Design review of the part built by this model. Coordinates are the model's own, in mm. A direction names the side the tool comes from. Coordinates: 2 decimals unless noted, no trailing zeros. Loops run counter-clockwise (first coordinate to the right, second up) from the corner with the lowest first, then second, coordinate; pieces in that order, holes last. Notation, with made-up numbers: (-16.75, 15) - (27.25, 15) arc R20 ccw to (27.25, 43) - close; hole circle Ø6 at (21, -12). An arc over 180 degrees is marked (long way). Return JSON: item names as keys, results as strings. Group by question number.
from build123d import *

# Parameters (mm, degrees)
SKETCH1_R                   = 3.175
BOSS_EXTRUDE1_DEPTH         = 12.7
SKETCH3_R                   = 83.82
SKETCH3_R_2                 = 81.9404
CUT_EXTRUDE1_DEPTH          = 6.35
CUT_EXTRUDE2_START          = -6.35
CUT_EXTRUDE2_OUTLINE_R      = 81.9404
CUT_EXTRUDE2_DEPTH          = 6.35
F_1_4_0_25_DIAMETER_HOLE1_D = 6.35
FILLET1_R                   = 6.35
CUT_EXTRUDE3_DEPTH          = 1047.720478305


# Read off the part's stored shape, not the designer's step: Cut-Extrude2
with BuildPart() as part:
    # Sketch1 → Boss-Extrude1 (new body)
    with BuildSketch(Plane.XZ.offset(-27489.985969718)):
        Polygon((556.409465543, 581.693641464), (28.480379396, 886.493641464), (-276.319620604, 358.564555317), (251.609465543, 53.764555317), align=None)
        with Locations((-206.925530091, 377.158645829)):
            Circle(SKETCH1_R, mode=Mode.SUBTRACT)
        with Locations((233.015375031, 123.158645829)):
            Circle(SKETCH1_R, mode=Mode.SUBTRACT)
        with Locations((487.015375031, 563.099550952)):
            Circle(SKETCH1_R, mode=Mode.SUBTRACT)
        with Locations((47.074469909, 817.099550952)):
            Circle(SKETCH1_R, mode=Mode.SUBTRACT)
        with BuildLine():
            Line((-37.632916951, 543.382053135), (-48.631439579, 549.732053135))
            Line((-48.631439579, 549.732053135), (-35.931439579, 571.729098391))
            Line((-35.931439579, 571.729098391), (-13.934394323, 559.029098391))
            Line((-13.934394323, 559.029098391), (-20.284394323, 548.030575763))
            ThreePointArc((-20.284394323, 548.030575763), (-27.995915078, 542.113317769), (-37.632916951, 543.382053135))
        make_face(mode=Mode.SUBTRACT)
        with BuildLine():
            Line((241.64492247, 646.10546044), (263.641967726, 633.40546044))
            Line((263.641967726, 633.40546044), (257.291967726, 622.406937812))
            ThreePointArc((257.291967726, 622.406937812), (249.580446971, 616.489679818), (239.943445098, 617.758415184))
            Line((239.943445098, 617.758415184), (228.94492247, 624.108415184))
            Line((228.94492247, 624.108415184), (241.64492247, 646.10546044))
        make_face(mode=Mode.SUBTRACT)
    extrude(amount=BOSS_EXTRUDE1_DEPTH)

    # Sketch3 → Cut-Extrude1 (cut)
    with BuildSketch(Plane.XZ.offset(-27489.985969718)):
        with Locations((140.04492247, 470.129098391)):
            Circle(SKETCH3_R)
        with Locations((140.04492247, 470.129098391)):
            Circle(SKETCH3_R_2, mode=Mode.SUBTRACT)
    extrude(amount=CUT_EXTRUDE1_DEPTH, mode=Mode.SUBTRACT)

    # Cut-Extrude2 outline → Cut-Extrude2 (cut)
    with BuildSketch(Plane(origin=(0, 27489.985969718, 0), x_dir=(1, 0, 0), z_dir=(0, 1, 0)).offset(CUT_EXTRUDE2_START)):
        with Locations((140.04492247, -470.129098391)):
            Circle(CUT_EXTRUDE2_OUTLINE_R)
        with BuildLine():
            ThreePointArc((74.203873091, -422.730325217), (99.48112247, -399.870535843), (131.916905483, -389.409690429))
            ThreePointArc((131.916905483, -389.409690429), (135.589601797, -390.547508644), (137.326798106, -393.977592825))
            ThreePointArc((137.326798106, -393.977592825), (140.04492247, -396.516851306), (142.763046834, -393.977592825))
            ThreePointArc((142.763046834, -393.977592825), (144.500243143, -390.547508644), (148.172939457, -389.409690429))
            ThreePointArc((148.172939457, -389.409690429), (180.60872247, -399.870535843), (205.885971849, -422.730325217))
            ThreePointArc((205.885971849, -422.730325217), (206.736940528, -426.479882633), (204.634998644, -429.699380858))
            ThreePointArc((204.634998644, -429.699380858), (203.794998475, -433.322974849), (207.353123009, -434.407310358))
            ThreePointArc((207.353123009, -434.407310358), (211.192261201, -434.196724402), (214.013988837, -436.808463603))
            ThreePointArc((214.013988837, -436.808463603), (221.17252247, -470.129098391), (214.013988837, -503.449733178))
            ThreePointArc((214.013988837, -503.449733178), (211.192261202, -506.06147238), (207.353123009, -505.850886424))
            ThreePointArc((207.353123009, -505.850886424), (203.794998475, -506.935221933), (204.634998644, -510.558815924))
            ThreePointArc((204.634998644, -510.558815924), (206.736940528, -513.778314149), (205.885971849, -517.527871565))
            ThreePointArc((205.885971849, -517.527871565), (180.60872247, -540.387660939), (148.172939457, -550.848506352))
            ThreePointArc((148.172939457, -550.848506352), (144.500243143, -549.710688138), (142.763046834, -546.280603957))
            ThreePointArc((142.763046834, -546.280603957), (140.04492247, -543.741345476), (137.326798106, -546.280603957))
            ThreePointArc((137.326798106, -546.280603957), (135.589601797, -549.710688138), (131.916905483, -550.848506352))
            ThreePointArc((131.916905483, -550.848506352), (99.48112247, -540.387660939), (74.203873091, -517.527871565))
            ThreePointArc((74.203873091, -517.527871565), (73.352904412, -513.778314149), (75.454846296, -510.558815924))
            ThreePointArc((75.454846296, -510.558815924), (76.294846465, -506.935221933), (72.736721931, -505.850886424))
            ThreePointArc((72.736721931, -505.850886424), (68.897583739, -506.06147238), (66.075856104, -503.449733178))
            ThreePointArc((66.075856104, -503.449733178), (58.91732247, -470.12909839), (66.075856104, -436.808463603))
            ThreePointArc((66.075856104, -436.808463603), (68.897583739, -434.196724402), (72.736721931, -434.407310358))
            ThreePointArc((72.736721931, -434.407310358), (76.294846465, -433.322974849), (75.454846296, -429.699380858))
            ThreePointArc((75.454846296, -429.699380858), (73.352904412, -426.479882633), (74.203873091, -422.730325217))
        make_face(mode=Mode.SUBTRACT)
    extrude(amount=CUT_EXTRUDE2_DEPTH, mode=Mode.SUBTRACT)

    # 1/4 (0.25) Diameter Hole1 (through all)
    with Locations(Plane(origin=(0, 27477.285969718, 0), x_dir=(-1, 0, 0), z_dir=(0, -1, 0))):
        with Locations((-276.56992247, -706.597334894), (-276.56992247, -233.660861887), (133.00507753, -470.129098391), (-140.04492247, -470.129098391)):
            Hole(F_1_4_0_25_DIAMETER_HOLE1_D / 2)

    # Fillet1
    fillet1_edges = [part.edges().sort_by_distance(p)[0] for p in [
        (-13.934394323, 27483.635969718, 559.029098391),
        (-35.931439579, 27483.635969718, 571.729098391),
        (-48.631439579, 27483.635969718, 549.732053135),
        (241.64492247, 27483.635969718, 646.10546044),
        (228.94492247, 27483.635969718, 624.108415184),
        (263.641967726, 27483.635969718, 633.40546044),
    ]]
    fillet(fillet1_edges, radius=FILLET1_R)

    # Sketch7 → Cut-Extrude3 (cut, through all)
    with BuildSketch(Plane(origin=(0, 27489.985969718, 0), x_dir=(1, 0, 0), z_dir=(0, 1, 0))):
        with BuildLine():
            Line((87.519099271, -555.383941842), (88.589697985, -541.194514974))
            ThreePointArc((88.589697985, -541.194514974), (90.165199445, -538.685494585), (93.125578624, -538.569119019))
            Line((93.125578624, -538.569119019), (98.706273756, -541.238167012))
            ThreePointArc((98.706273756, -541.238167012), (98.923894245, -541.352808536), (99.131986961, -541.483952646))
            Line((99.131986961, -541.483952646), (104.233797894, -544.982452404))
            ThreePointArc((104.233797894, -544.982452404), (105.613203287, -547.604403762), (104.228078621, -550.223338244))
            Line((104.228078621, -550.223338244), (92.474973845, -558.245217361))
            ThreePointArc((92.474973845, -558.245217361), (89.0976004, -558.372448725), (87.519099271, -555.383941842))
        make_face()
        with BuildLine():
            Line((92.474973844, -382.01297942), (104.228078621, -390.034858537))
            ThreePointArc((104.228078621, -390.034858537), (105.613203286, -392.65379302), (104.233797893, -395.275744378))
            Line((104.233797893, -395.275744378), (99.131986961, -398.774244135))
            ThreePointArc((99.131986961, -398.774244135), (98.923894245, -398.905388245), (98.706273756, -399.020029769))
            Line((98.706273756, -399.020029769), (93.125578624, -401.689077763))
            ThreePointArc((93.125578624, -401.689077763), (90.165199444, -401.572702196), (88.589697984, -399.063681808))
            Line((88.589697984, -399.063681808), (87.519099271, -384.874254939))
            ThreePointArc((87.519099271, -384.874254939), (89.0976004, -381.885748056), (92.474973844, -382.01297942))
        make_face()
        with BuildLine():
            Line((240.140694294, -472.990373909), (227.316990804, -479.157921661))
            ThreePointArc((227.316990804, -479.157921661), (224.356364679, -479.048007567), (222.775390892, -476.542431776))
            Line((222.775390892, -476.542431776), (222.296506693, -470.374884024))
            ThreePointArc((222.296506693, -470.374884024), (222.28697892, -470.12909839), (222.296506693, -469.883312757))
            Line((222.296506693, -469.883312757), (222.775390892, -463.715765005))
            ThreePointArc((222.775390892, -463.715765005), (224.356364679, -461.210189214), (227.316990804, -461.10027512))
            Line((227.316990804, -461.10027512), (240.140694294, -467.267822872))
            ThreePointArc((240.140694294, -467.267822872), (241.939566609, -470.12909839), (240.140694294, -472.990373909))
        make_face()
    extrude(amount=-CUT_EXTRUDE3_DEPTH, mode=Mode.SUBTRACT)


solid = part.part
Item 1: Add section C-C (x = 6). State the section outline as (y, z) points.
Item 2: To check wall thickness, follow line 1 (X direction, y = 27483, z = 548); line 2 (X direction, y = 27489.75, z = 440); line 3 (X direction, y = 27478.75, z = 619). State the ranges of each line that lie inside material, in increasing order. Write a range as from..to.
Item 3: Add section A-A (y = 27485.75). Give the number of separate pieces and of enclosed holes in the cut face, then the cut area to 3 significant figures.
Item 4: Add section B-B (z = 140). State the section outline as (x, y) points.
Item 5: For faces 5 (the face through (-16.05, 27483.72, 208.3)), 6 (the face through (180.99, 27486.86, 396.99)), list the 3-axis set-ups (+Z, -Z, +X, -X, +Y, -Y) from which the entire face can be reached by the end or side of a thin tool; tool diameter is ignored.
Item 6: Draft analysis for pull direction X (two halves, no side actions). For faces 1 (the face through (56.232, 27486.855, 471.244)), 2 (the face through (139, 27489.986, 453)), 3 (the face through (-121.8, 27483.7, 626.2)), 4 (the face through (99.07, 27486.77, 400.11)), state which applies: pulls with the +X half, pulls with the -X half, needs draft (parallel to the pull), parting line crosses it, or undercut.
Item 7: For P1, Ø10, axis at x = 233.02, z = 123.16, coming from the +Y side; P2, Ø2, axis at x = 463, y = 27488.5, coming from the +Z side; P3, Ø2, axis at x = 386.5, y = 27488, coming from the -Z side; P4, Ø1.5, axis at y = 27485.5, z = 347.5, coming from the +X side, all flat-tipped, find the tip position at first contact; note any pin that passes through.
Answers below:
{
 "1": {"outline": "(27477.29, 195.57) - (27489.99, 195.57) - (27489.99, 847.56) - (27477.29, 847.56) - close"},
 "2": {"line 1": "x = -166.95..-44.84, -20.3..88.08, 105.59..536.96", "line 2": "x = -229.3..61.83, 64.72..215.37, 218.26..474.6", "line 3": "x = -125.96..237.79, 254.42..491.79"},
 "3": {"separate pieces": "2", "enclosed holes": "11", "area": "368,000 mm^2"},
 "4": {"outline": "(102.25, 27477.29) - (301.4, 27477.29) - (301.4, 27489.99) - (102.25, 27489.99) - close"},
 "5": {"face 5": "-Z, -X, +Y, -Y", "face 6": "+Y"},
 "6": {"face 1": "undercut", "face 2": "needs draft", "face 3": "pulls with the -X half", "face 4": "undercut"},
 "7": {"P1": "stops at y = 27489.99", "P2": "stops at z = 636.2", "P3": "stops at z = 285.67", "P4": "stops at x = 421.63"}
}
